```python
from build123d import *

# Parameters (mm, degrees)
BOSS_EXTRUDE1_DEPTH = 100
CUT_EXTRUDE1_DEPTH  = 100
CUT_EXTRUDE3_DEPTH  = 100
FILLET1_R           = 0.25
CUT_EXTRUDE4_DEPTH  = 100
SKETCH6_R           = 3.5
CUT_EXTRUDE5_DEPTH  = 1
SKETCH7_R           = 3.5
CUT_EXTRUDE6_DEPTH  = 10.24


with BuildPart() as part:
    # Sketch1 → Boss-Extrude1 (new body)
    with BuildSketch(Plane.XY):
        Polygon((-93.7, 0), (93.7, 0), (0, 100), align=None)
    extrude(amount=BOSS_EXTRUDE1_DEPTH)

    # Sketch3 → Cut-Extrude1 (cut)
    with BuildSketch(Plane(origin=(0, 0, 0), x_dir=(1, 0, 0), z_dir=(0, 1, 0))):
        with BuildLine():
            Line((86.649916098, -18.521939898), (93.7, -26.944779698))
            Line((93.7, -26.944779698), (117.286189742, 18.149796591))
            ThreePointArc((117.286189742, 18.149796591), (0, 220), (-117.286189742, 18.149796591))
            Line((-117.286189742, 18.149796591), (-93.7, -26.944779698))
            Line((-93.7, -26.944779698), (-86.649916098, -18.521939898))
            ThreePointArc((-86.649916098, -18.521939898), (0, -50), (86.649916098, -18.521939898))
        make_face()
    extrude(amount=CUT_EXTRUDE1_DEPTH, mode=Mode.SUBTRACT)

    # Sketch4 → Cut-Extrude3 (cut)
    with BuildSketch(Plane(origin=(0, 0, 0), x_dir=(1, 0, 0), z_dir=(0, 1, 0))):
        with BuildLine():
            Line((-145, 85), (-145, -157.27076369))
            Line((-145, -157.27076369), (195.83768652, -157.27076369))
            Line((195.83768652, -157.27076369), (144.517709557, 73.183417402))
            ThreePointArc((144.517709557, 73.183417402), (-5.913210388, -59.879377217), (-145, 85))
        make_face()
    extrude(amount=CUT_EXTRUDE3_DEPTH, mode=Mode.SUBTRACT)

    # Fillet1
    fillet1_edges = [part.edges().sort_by_distance(p)[0] for p in [
        (0, 100, 55),
    ]]
    fillet(fillet1_edges, radius=FILLET1_R)

    # Sketch5 → Cut-Extrude4 (cut)
    with BuildSketch(Plane.XY):
        with BuildLine():
            ThreePointArc((1.75, 70.74941109), (-0.695889742, 72.355100184), (-1.196557105, 69.472402439))
            Line((-1.196557105, 69.472402439), (0, 70.74941109))
            Line((0, 70.74941109), (1.196557105, 69.472402439))
            ThreePointArc((1.196557105, 69.472402439), (1.605689094, 70.053521348), (1.75, 70.74941109))
        make_face()
        with BuildLine():
            Line((0, 70.74941109), (-1.196557105, 69.472402439))
            ThreePointArc((-1.196557105, 69.472402439), (0, 68.99941109), (1.196557105, 69.472402439))
            Line((1.196557105, 69.472402439), (0, 70.74941109))
        make_face()
        with BuildLine():
            ThreePointArc((46.355641086, 21.27700865), (45.946509097, 20.695889742), (45.802198191, 20))
            Line((45.802198191, 20), (47.552198191, 20))
            Line((47.552198191, 20), (46.355641086, 21.27700865))
        make_face()
        with BuildLine():
            Line((47.552198191, 20), (45.802198191, 20))
            ThreePointArc((45.802198191, 20), (47.552198191, 18.25), (49.302198191, 20))
            ThreePointArc((49.302198191, 20), (48.248087933, 21.605689094), (46.355641086, 21.27700865))
            Line((46.355641086, 21.27700865), (47.552198191, 20))
        make_face()
        with BuildLine():
            Line((-46.355641086, 21.27700865), (-47.552198191, 20))
            Line((-47.552198191, 20), (-45.802198191, 20))
            ThreePointArc((-45.802198191, 20), (-45.946509097, 20.695889742), (-46.355641086, 21.27700865))
        make_face()
        with BuildLine():
            Line((-45.802198191, 20), (-47.552198191, 20))
            Line((-47.552198191, 20), (-46.355641086, 21.27700865))
            ThreePointArc((-46.355641086, 21.27700865), (-49.157887285, 19.304110258), (-45.802198191, 20))
        make_face()
    extrude(amount=CUT_EXTRUDE4_DEPTH, mode=Mode.SUBTRACT)

    # Sketch6 → Cut-Extrude5 (cut)
    with BuildSketch(Plane.XY.offset(60)):
        with Locations((0, 70.74941109)):
            Circle(SKETCH6_R)
    extrude(amount=-CUT_EXTRUDE5_DEPTH, mode=Mode.SUBTRACT)

    # Sketch7 → Cut-Extrude6 (cut)
    with BuildSketch(Plane.XY.offset(60)):
        with Locations((-47.552198191, 20)):
            Circle(SKETCH7_R)
        with Locations((47.552198191, 20)):
            Circle(SKETCH7_R)
    extrude(amount=-CUT_EXTRUDE6_DEPTH, mode=Mode.SUBTRACT)


solid = part.part
```
Model file for the job. Use its own axes, mm. A direction names the side the tool comes from. Coordinates: 2 decimals unless noted, no trailing zeros. Order: outer loops, then holes, each group sorted by start corner. A loop starts at its lowest first (then second) coordinate and runs counter-clockwise, first axis right, second up. Notation, with made-up numbers: (83.5, 75.25) -> (139.5, 75.25) arc R27 ccw to (139.5, 104.25) -> close; hole circle Ø9 at (79, 17.5). An arc over 180 degrees is marked (long way). Answer as a JSON object with one key per item and string values. Group by question number.
1) Drill centre lines: L1, parallel to Y at x = 0, z = 59.5; L2, parallel to X at y = 20, z = 51.25; L3, parallel to X at y = 10, z = 34.5. Where is each one in solid material? Low to high.
2) Flat gauge pins, fed straight in: pin 1 (6.5 mm diameter, centred on x = 0, y = 70.75, fed in from -Z); pin 2 (1.5 mm diameter, centred on y = 78, z = 48.5, fed in from -X); pin 3 (12 mm diameter, centred on y = 38, z = 29, fed in from -X); pin 4 (3 mm diameter, centred on y = 88, z = 52, fed in from -X). Where does each tip first touch, or does it go through?
3) Cut at A-A, the plane z = 47. Write the cut outline in (x, y), then the cut area to 3 significant figures.
4) Cut at C-C, the plane y = 81.5. Write the cut outline in (x, z).
5) Cut at D-D, the plane x = -19.5. Write the cut outline in (y, z), then the cut area to 3 significant figures.
6) Pull direction Z, two halves, no side cores. Call faces 3 (the face through (-1.317, 27.046, 49.994)), 4 (the face through (46.84, 50.01, 42.24)), 5 (the face through (1.415, 27.046, 59.993)): +Z half, -Z half, draft (parallel to the pull), parting line (faces both ways), or undercut.
7) Which spindle directions (+Z, -Z, +X, -X, +Y, -Y) get a long thin tool onto all of the face, cutting with end or side? Do faces 1 (the face through (44.056, 20.154, 51.112)), 2 (the face through (-89.191, 2.873, 21.558)). Say none if no direction does.
8) Cut at B-B, the plane z = 31.5. Write the cut outline in (x, y), then the cut area to 3 significant figures.
Check values:
{
 "1": {"L1": "y = 0 to 67.25, 74.25 to 99.88", "L2": "x = -44.05 to 44.05", "L3": "x = -82.13 to -62.81, 62.81 to 82.13"},
 "2": {"pin 1": "stops at z = 49.96", "pin 2": "stops at x = -21.32", "pin 3": "passes through", "pin 4": "stops at x = -12.65"},
 "3": {"outline": "(-60.01, 0) -> (-28.3, 0) -> (-28.3, 69.8) -> (-60.01, 35.96) -> close; (28.3, 0) -> (60.01, 0) -> (60.01, 35.96) -> (28.3, 69.8) -> close; hole circle Ø3.5 at (-47.55, 20); hole circle Ø3.5 at (47.55, 20)", "area": "3,330 mm²"},
 "4": {"outline": "(-17.33, 48.88) arc R135 cw to (17.33, 48.88) -> (17.33, 58.96) arc R145 ccw to (-17.33, 58.96) -> close"},
 "5": {"outline": "(0, 48.58) -> (79.19, 48.58) -> (79.19, 58.68) -> (0, 58.68) -> close", "area": "800 mm²"},
 "6": {"face 3": "-Z half", "face 4": "draft", "face 5": "+Z half"},
 "7": {"face 1": "+Z", "face 2": "-Z, -X, +Y, -Y"},
 "8": {"outline": "(-86.33, 0) -> (-68.21, 0) -> (-68.21, 27.2) -> (-86.33, 7.87) -> close; (68.21, 0) -> (86.33, 0) -> (86.33, 7.87) -> (68.21, 27.2) -> close", "area": "635 mm²"}
}
